The figure shows three views and two pictorial views of one solid part (mm, origin at its lowest corner). Answer the questions. A direction names the side the tool comes from. Coordinates: 2 decimals unless noted, no trailing zeros. Order: outer loops, then holes, each group sorted by start corner. A loop starts at its lowest first (then second) coordinate and runs counter-clockwise, first axis right, second up. Notation, with made-up numbers: (-6.5, 25.5) -> (43.5, 25.5) arc R15 cw to (43.5, 45.5) -> close; hole circle Ø7 at (58, 37.5). An arc over 180 degrees is marked (long way). Return JSON: item names as keys, results as strings.
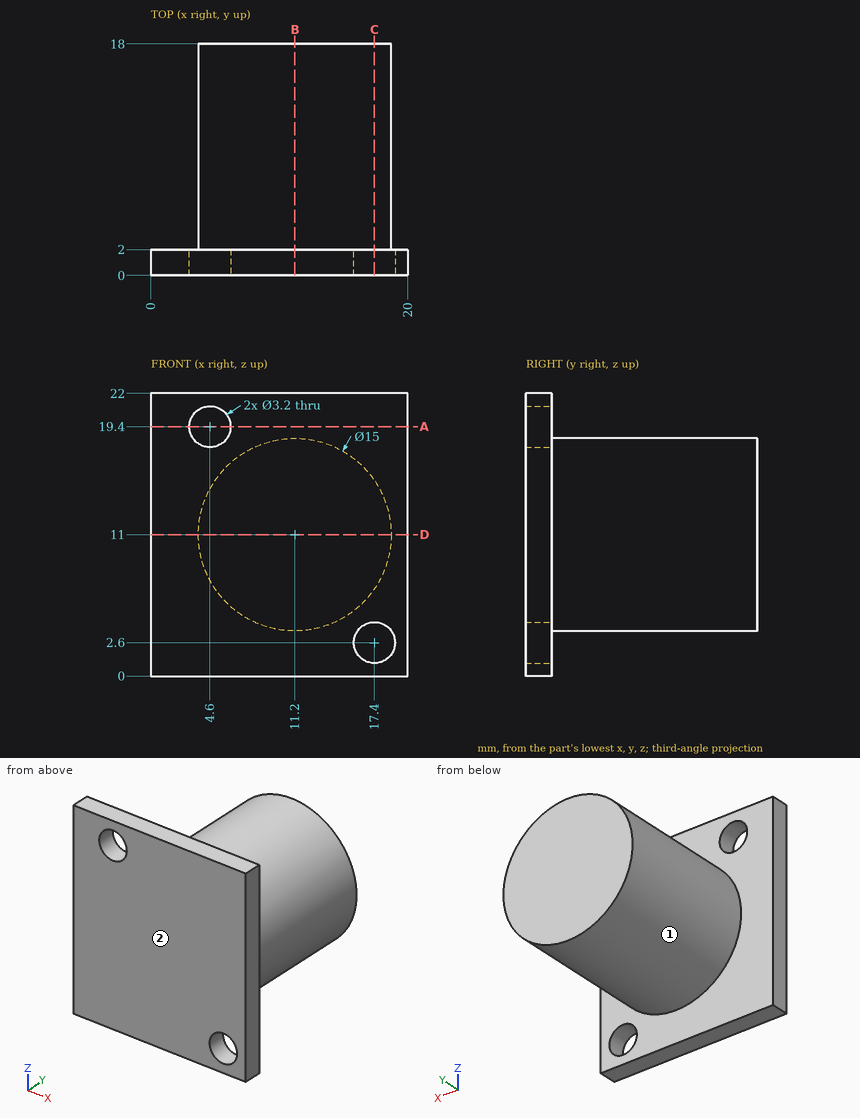
1. The part is cut by section C-C on x = 17.4. Give the vertices of the cut face in (y, z), and give its area (3 significant figures).
Answer block:
{"outline": "(0, 0) -> (2, 0) -> (2, 1) -> (0, 1) -> close; (0, 4.2) -> (2, 4.2) -> (2, 6.78) -> (18, 6.78) -> (18, 15.22) -> (2, 15.22) -> (2, 22) -> (0, 22) -> close", "area": "173 mm2"}
2. The part is cut by section B-B on x = 11.2. Give the vertices of the cut face in (y, z), and give its area (3 significant figures).
Answer block:
{"outline": "(0, 0) -> (2, 0) -> (2, 3.5) -> (18, 3.5) -> (18, 18.5) -> (2, 18.5) -> (2, 22) -> (0, 22) -> close", "area": "284 mm2"}
3. Each of these flat-tipped pins is pushed along its axis until it touches: pin 1 Ø1 at (x, y) = (8, 9) entering from +Z; pin 2 Ø2 at (x, y) = (15.5, 8) entering from +Z (3 decimals); pin 3 Ø5 at (x, z) = (4.6, 19.4) entering from +Y. Where does it stop, or does it pass through?
Answer block:
{"pin 1": "stops at z = 18", "pin 2": "stops at z = 17.735", "pin 3": "stops at y = 2"}
4. The part is cut by section D-D on z = 11. Give the vertices of the cut face in (x, y), and give its area (3 significant figures).
Answer block:
{"outline": "(0, 0) -> (20, 0) -> (20, 2) -> (18.7, 2) -> (18.7, 18) -> (3.7, 18) -> (3.7, 2) -> (0, 2) -> close", "area": "280 mm2"}
5. Consider line 1 (X direction, y = 0.6, z = 19.4); line 2 (Z direction, x = 4.6, y = 0.9); line 3 (X direction, y = 1.15, z = 2.6). Determine where each line is inside the solid, lowest interval first. Write a range as from..to.
Answer block:
{"line 1": "x = 0..3, 6.2..20", "line 2": "z = 0..17.8, 21..22", "line 3": "x = 0..15.8, 19..20"}
6. For the marked faces 1 and 2, determine the directions among +Z, -Z, +X, -X, +Y, -Y from which every point of the face is accessible in a straight line to the end or side of a thin tool.
Answer block:
{"face 1": "+Y", "face 2": "+Z, -Z, +X, -X, -Y"}
7. The part is cut by section A-A on z = 19.4. Give the vertices of the cut face in (x, y), and give its area (3 significant figures).
Answer block:
{"outline": "(0, 0) -> (3, 0) -> (3, 2) -> (0, 2) -> close; (6.2, 0) -> (20, 0) -> (20, 2) -> (6.2, 2) -> close", "area": "33.6 mm2"}
